Part print with two shaded views. Sizes in mm from the minimum x, y, z corner. A direction names the side the tool comes from. Round coordinates to 2 decimals unless told otherwise and drop trailing zeros. Loops run counter-clockwise (first coordinate to the right, second up) from the corner with the lowest first, then second, coordinate; pieces in that order, holes last. Notation, with made-up numbers: (-1, -17.75) - (28, -17.75) arc R17 cw to (28, -6.75) - close; hole circle Ø2 at (6, 87.5). An arc over 180 degrees is marked (long way). Use a Markdown table: item, result.
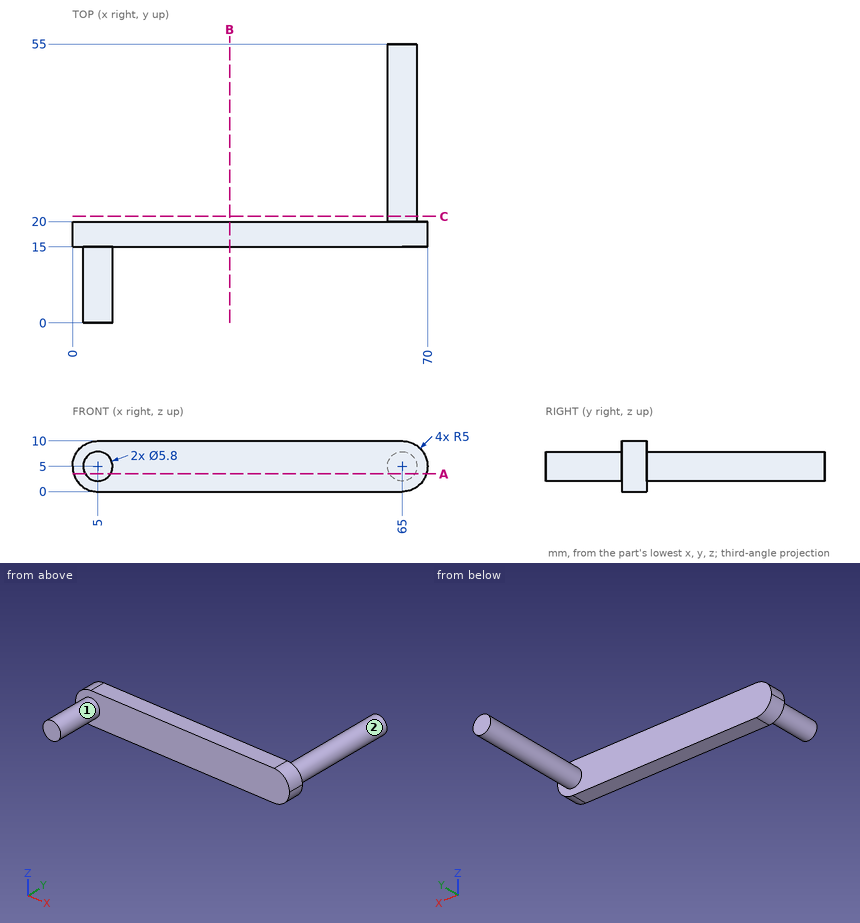
Q1. Drop flat-ended pins along their axis: pin 1 (3 mm diameter, centred on x = 47.5, z = 3, fed in from +Y); pin 2 (3 mm diameter, centred on y = 6.5, z = 7, fed in from +X); pin 3 (4 mm diameter, centred on y = 27.5, z = 7, fed in from +X). Give the stop position or say it passes through.
Results found:
| item | result |
|---|---|
| pin 1 | stops at y = 20 |
| pin 2 | stops at x = 7.86 |
| pin 3 | stops at x = 67.9 |
Q2. Cut at B-B, the plane x = 31. List the corners of the cut face in (y, z), plus the area to 3 significant figures.
Results found:
| item | result |
|---|---|
| outline | (15, 0) - (20, 0) - (20, 10) - (15, 10) - close |
| area | 50.0 mm2 |
Q3. Cut at A-A, the plane z = 3.5. List the corners of the cut face in (x, y), plus the area to 3 significant figures.
Results found:
| item | result |
|---|---|
| outline | (0.23, 15) - (2.52, 15) - (2.52, 0) - (7.48, 0) - (7.48, 15) - (69.77, 15) - (69.77, 20) - (67.48, 20) - (67.48, 55) - (62.52, 55) - (62.52, 20) - (0.23, 20) - close |
| area | 596 mm2 |
Q4. Probe line 1 (Y direction, x = 56, z = 8); line 2 (X direction, y = 42, z = 7.25); line 3 (X direction, y = 20.5, z = 5.5). List the from-to ranges inside material, lowest first.
Results found:
| item | result |
|---|---|
| line 1 | y = 15 to 20 |
| line 2 | x = 63.17 to 66.83 |
| line 3 | x = 62.14 to 67.86 |
Q5. Which spindle directions (+Z, -Z, +X, -X, +Y, -Y) get a long thin tool onto all of the face, cutting with end or side? Do the marked faces 1 and 2. Say none if no direction does.
Results found:
| item | result |
|---|---|
| face 1 | -Y |
| face 2 | +Y |
Q6. Cut at C-C, the plane y = 21. List the corners of the cut face in (x, z), plus the area to 3 significant figures.
Results found:
| item | result |
|---|---|
| outline | circle Ø5.8 at (65, 5) |
| area | 26.4 mm2 |
